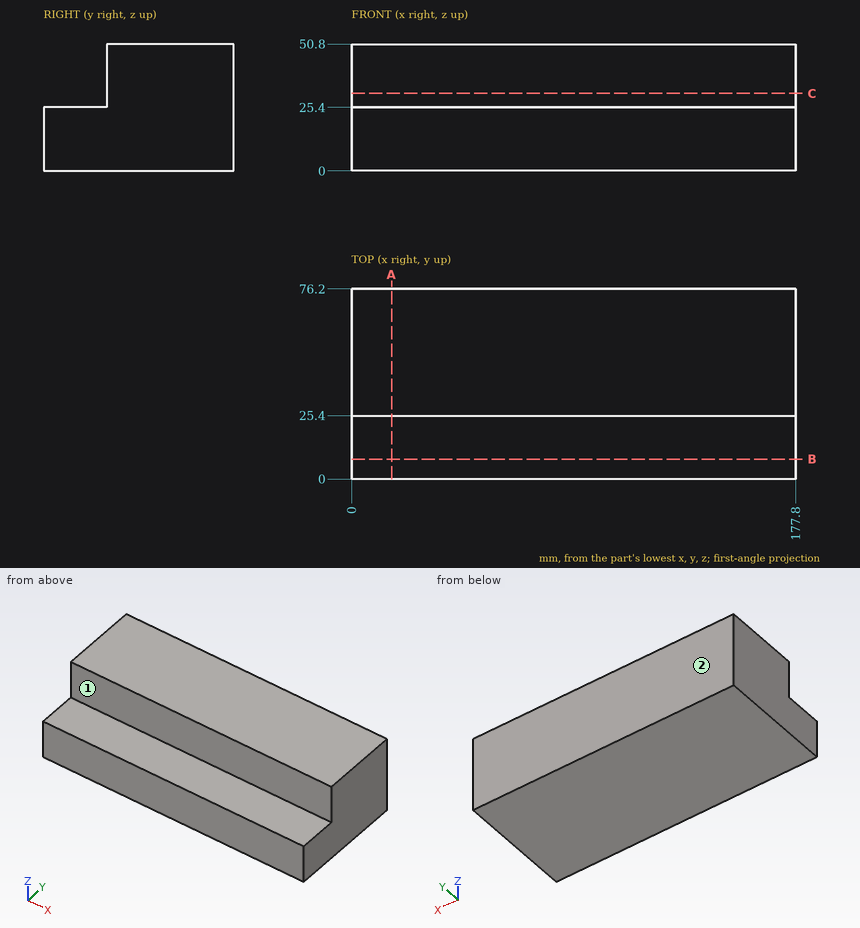
Verification items for this drawing (mm, ordinates from the low corner). A direction names the side the tool comes from. Coordinates: 2 decimals unless noted, no trailing zeros. Order: outer loops, then holes, each group sorted by start corner. A loop starts at its lowest first (then second) coordinate and runs counter-clockwise, first axis right, second up. Notation, with made-up numbers: (15, 16) -> (36, 16) arc R16 cw to (36, 38) -> close; hole circle Ø4 at (71.25, 71). An arc over 180 degrees is marked (long way). Answer as CSV lines item,"result". Start each with the question number.
1) Set-up check for the marked faces 1 and 2: record each of +Z, -Z, +X, -X, +Y, -Y from which the full face is reachable in a straight line by a thin tool's end or side.
2) Cross-section at A-A, the plane x = 16. Record the boundary of the cut face in (y, z), then the cut area to 3 significant figures.
3) Cross-section at B-B, the plane y = 8. Record the boundary of the cut face in (x, z), then the cut area to 3 significant figures.
4) Gauge pin test, flat ends, axial feed: pin 1 Ø8 at (x, y) = (49, 9) entering from +Z; pin 2 Ø20.5 at (x, z) = (100.5, 43) entering from -Y. Record the tip position at first contact, or that the pin passes through.
5) Cross-section at C-C, the plane z = 31. Record the boundary of the cut face in (x, y), then the cut area to 3 significant figures.
6) Material ranges on L1, parallel to Y at x = 102, z = 27; L2, parallel to Z at x = 53.5, y = 19.5, recorded low to high. Write a range as [from, to].
Conclusion:
1,face 1,"+Z, +X, -X, -Y"
1,face 2,"+Z, -Z, +X, -X, +Y"
2,outline,"(0, 0) -> (76.2, 0) -> (76.2, 50.8) -> (25.4, 50.8) -> (25.4, 25.4) -> (0, 25.4) -> close"
2,area,"3,230 mm²"
3,outline,"(0, 0) -> (177.8, 0) -> (177.8, 25.4) -> (0, 25.4) -> close"
3,area,"4,520 mm²"
4,pin 1,"stops at z = 25.4"
4,pin 2,"stops at y = 25.4"
5,outline,"(0, 25.4) -> (177.8, 25.4) -> (177.8, 76.2) -> (0, 76.2) -> close"
5,area,"9,030 mm²"
6,L1,"y = [25.4, 76.2]"
6,L2,"z = [0, 25.4]"
